from build123d import *

# Parameters (mm, degrees)
F1_START = 50
F0_R     = 21.5
F0_R_2   = 16.5
F1_DEPTH = 200
F2_DEPTH = 70
F3_R     = 6.5
F4_DEPTH = 42
F4_TAPER = 8
F5_R     = 20.2793939239


with BuildPart() as f1:
    # F0 (on Top) → F1 (new body)
    with BuildSketch(Plane.XY.offset(F1_START)):
        with Locations((27.2554606199, 24.6764030308)):
            Circle(F0_R)
        with Locations((27.2554606199, 24.6764030308)):
            Circle(F0_R_2, mode=Mode.SUBTRACT)
        with Locations((27.2554606199, 24.6764030308)):
            Circle(F0_R_2)
    extrude(amount=F1_DEPTH)

    # F0 (on Top) → F2 (cut)
    with BuildSketch(Plane.XY):
        with Locations((27.2554606199, 24.6764030308)):
            Circle(F0_R)
        with Locations((27.2554606199, 24.6764030308)):
            Circle(F0_R_2, mode=Mode.SUBTRACT)
    extrude(amount=F2_DEPTH, mode=Mode.SUBTRACT)

    # F3 (on face) → F4 (join)
    with BuildSketch(Plane(origin=(0, 0, 50), x_dir=(1, 0, 0), z_dir=(0, 0, -1))):
        with Locations((27.2554606199, -24.6764030308)):
            Circle(F3_R)
    extrude(amount=F4_DEPTH, taper=F4_TAPER)

    # F5
    f5_edges = [f1.edges().sort_by_distance(p)[0] for p in [
        (5.755461, 24.676403, 250),
    ]]
    fillet(f5_edges, radius=F5_R)


solid = f1.part
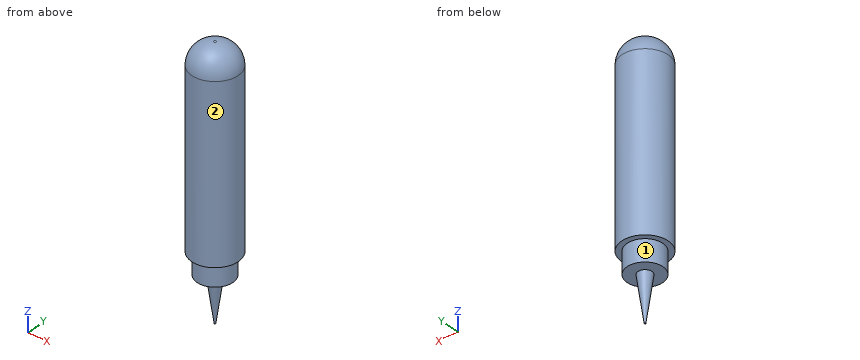
Source: CAD feature listing. Evaluate the final solid. Frame: model axes, mm. Face numbers are marked on the shaded views. A direction names the side the tool comes from. Coordinates: 2 decimals unless noted, no trailing zeros. Loops run counter-clockwise (first coordinate to the right, second up) from the corner with the lowest first, then second, coordinate; pieces in that order, holes last. Notation, with made-up numbers: (10, 62.5) - (39, 62.5) arc R19 cw to (39, 71.5) - close; hole circle Ø5 at (28, -3.75). An arc over 180 degrees is marked (long way). Return JSON: item names as keys, results as strings.
Q1. Section B-B, the plane z = 25. Return loops of the section in (x, y).
Results:
{"outline": "circle Ø5.97 at (27.26, 24.68)"}
Q2. Section A-A, the plane z = 53. Return loops of the section in (x, y), plus the area to 3 significant figures.
Results:
{"outline": "circle Ø33 at (27.26, 24.68)", "area": "855 mm2"}
Q3. Access query for the marked faces 1 and 2. Directions: +Z, -Z, +X, -X, +Y, -Y. A direction counts if a zero-diameter tool reaches every point of the face in a straight line with its end or side. Return the directions, or none.
Results:
{"face 1": "-Z", "face 2": "+Z, -Z"}
Q4. Contact query for flat-ended pins moving along their axis: P1, Ø1.5, axis at y = 33.5, z = 79.5, coming from the +X side; P2, Ø8, axis at y = 30.5, z = 68.5, coming from the +X side; P3, Ø2, axis at x = 24.5, y = 38.5, coming from the -Z side. Output: stop coordinate, or through.
Results:
{"P1": "x = 47.18", "P2": "x = 48.65", "P3": "z = 50"}
Q5. Material intervals for line 1 along X through (y, z) = (36.5, 236.5); line 2 along X through (y, z) = (40.5, 152.5); line 3 along Y through (x, z) = (26.5, 22.5), sorted ascending.
Results:
{"line 1": "10.71 to 43.8", "line 2": "12.7 to 41.81", "line 3": "22.15 to 27.2"}
